Read the model definition and answer for the solid it produces. Units are mm, in the model's axes. A direction names the side the tool comes from. Round coordinates to 2 decimals unless told otherwise and drop trailing zeros. Write each loop counter-clockwise with the first axis right and the second up, starting at its lowest first coordinate (ties: lowest second). Pieces come first, ordered by that corner, then holes. Notation, with made-up numbers: (63.25, -11.5) - (69.25, -11.5) arc R17 ccw to (69.25, 18.5) - close; hole circle Ø9 at (1, -7). An arc over 180 degrees is marked (long way). Use one line per item in the form item = value. Start each with the question number.
1) For a pull along X with two mould halves and no side action, classify faces 1 (the face through (7.5, 0, 4)), 2 (the face through (-6.7, -1, 4)), 3 (the face through (0, -1, 1)), 4 (the face through (0.1, 3.9, 4.5)) as released by +X, released by -X, zero draft, split by the parting line, or undercut.
2) This flat-tipped pin is pushed along its axis until it touches: pin 1 (0.5 mm diameter, centred on x = -3.5, z = 5.5, fed in from +Y). Where does it stop, or does it pass through?
3) Consider line 1 along X through (y, z) = (2, 6); line 2 along X through (y, z) = (-0.5, 4.5); line 3 along Y through (x, z) = (1, 3.5). Determine where each line is inside the solid, lowest interval first. Write a range as from..to.
4) The part is cut by section D-D, the plane z = 5.75. Give the vertices of the cut face in (x, y), plus the area to 3 significant figures.
5) The part is cut by section C-C, the plane z = 2.5. Give the vertices of the cut face in (x, y), plus the area to 3 significant figures.
6) For faces 5 (the face through (0, 3.5, 1)), 6 (the face through (0, -3.5, 4)), 7 (the face through (-5.7, 2, 4)), 8 (the face through (-0.1, 3.5, 5.5)), 9 (the face through (-0.1, 3.5, 7.5)), determine the directions among +Z, -Z, +X, -X, +Y, -Y from which every point of the face is accessible in a straight line to the end or side of a thin tool.
7) The part is cut by section B-B, the plane x = -3.5. Give the vertices of the cut face in (y, z).
8) The part is cut by section A-A, the plane y = -1.5. Give the vertices of the cut face in (x, z).
from build123d import *

# Parameters (mm, degrees)
F0_W     = 15
F0_H     = 7
F1_DEPTH = 1
F2_W     = 15
F2_H     = 7
F3_DEPTH = 7
F4_W     = 15
F4_H     = 1
F5_DEPTH = 0.4


with BuildPart() as f1:
    # F0 (on Top) → F1 (new body)
    with BuildSketch(Plane.XY):
        Rectangle(F0_W, F0_H)
    extrude(amount=F1_DEPTH)

    # F2 (on face) → F3 (join)
    with BuildSketch(Plane.XY.offset(1)):
        Rectangle(F2_W, F2_H)
        Polygon((-6.7, -2.7), (-6.7, 1.7), (-5.7, 1.7), (-5.7, 2.7), (-3.7, 2.7), (-3.7, 1.7), (3.7, 1.7), (3.7, 2.7), (5.7, 2.7), (5.7, 1.7), (6.7, 1.7), (6.7, -2.7), align=None, mode=Mode.SUBTRACT)
    extrude(amount=F3_DEPTH)

    # F4 (on face) → F5 (join)
    with BuildSketch(Plane(origin=(0, 3.5, 0), x_dir=(-1, 0, 0), z_dir=(0, 1, 0))):
        with Locations((0, 6.5)):
            Rectangle(F4_W, F4_H)
        with Locations((0, 4.5)):
            Rectangle(F4_W, F4_H)
        with Locations((0, 2.5)):
            Rectangle(F4_W, F4_H)
    extrude(amount=F5_DEPTH)


solid = f1.part
Geometry results:
q1.face_1 = released by +X
q1.face_2 = undercut
q1.face_3 = undercut
q1.face_4 = zero draft
q2.pin_1 = 3.5
q3.line_1 = -7.5..-5.7, -3.7..3.7, 5.7..7.5
q3.line_2 = -7.5..-6.7, 6.7..7.5
q3.line_3 = -3.5..-2.7, 1.7..3.5
q4.outline = (-7.5, -3.5) - (7.5, -3.5) - (7.5, 3.5) - (-7.5, 3.5) - close; hole (-6.7, -2.7) - (6.7, -2.7) - (6.7, 1.7) - (5.7, 1.7) - (5.7, 2.7) - (3.7, 2.7) - (3.7, 1.7) - (-3.7, 1.7) - (-3.7, 2.7) - (-5.7, 2.7) - (-5.7, 1.7) - (-6.7, 1.7) - close
q4.area = 42.0 mm2
q5.outline = (-7.5, -3.5) - (7.5, -3.5) - (7.5, 3.9) - (-7.5, 3.9) - close; hole (-6.7, -2.7) - (6.7, -2.7) - (6.7, 1.7) - (5.7, 1.7) - (5.7, 2.7) - (3.7, 2.7) - (3.7, 1.7) - (-3.7, 1.7) - (-3.7, 2.7) - (-5.7, 2.7) - (-5.7, 1.7) - (-6.7, 1.7) - close
q5.area = 48.0 mm2
q6.face_5 = -Z, +X, -X, +Y
q6.face_6 = +Z, -Z, +X, -X, -Y
q6.face_7 = +Z
q6.face_8 = +X, -X, +Y
q6.face_9 = +Z, +X, -X, +Y
q7.outline = (-3.5, 0) - (3.5, 0) - (3.5, 2) - (3.9, 2) - (3.9, 3) - (3.5, 3) - (3.5, 4) - (3.9, 4) - (3.9, 5) - (3.5, 5) - (3.5, 6) - (3.9, 6) - (3.9, 7) - (3.5, 7) - (3.5, 8) - (1.7, 8) - (1.7, 1) - (-2.7, 1) - (-2.7, 8) - (-3.5, 8) - close
q8.outline = (-7.5, 0) - (7.5, 0) - (7.5, 8) - (6.7, 8) - (6.7, 1) - (-6.7, 1) - (-6.7, 8) - (-7.5, 8) - close
